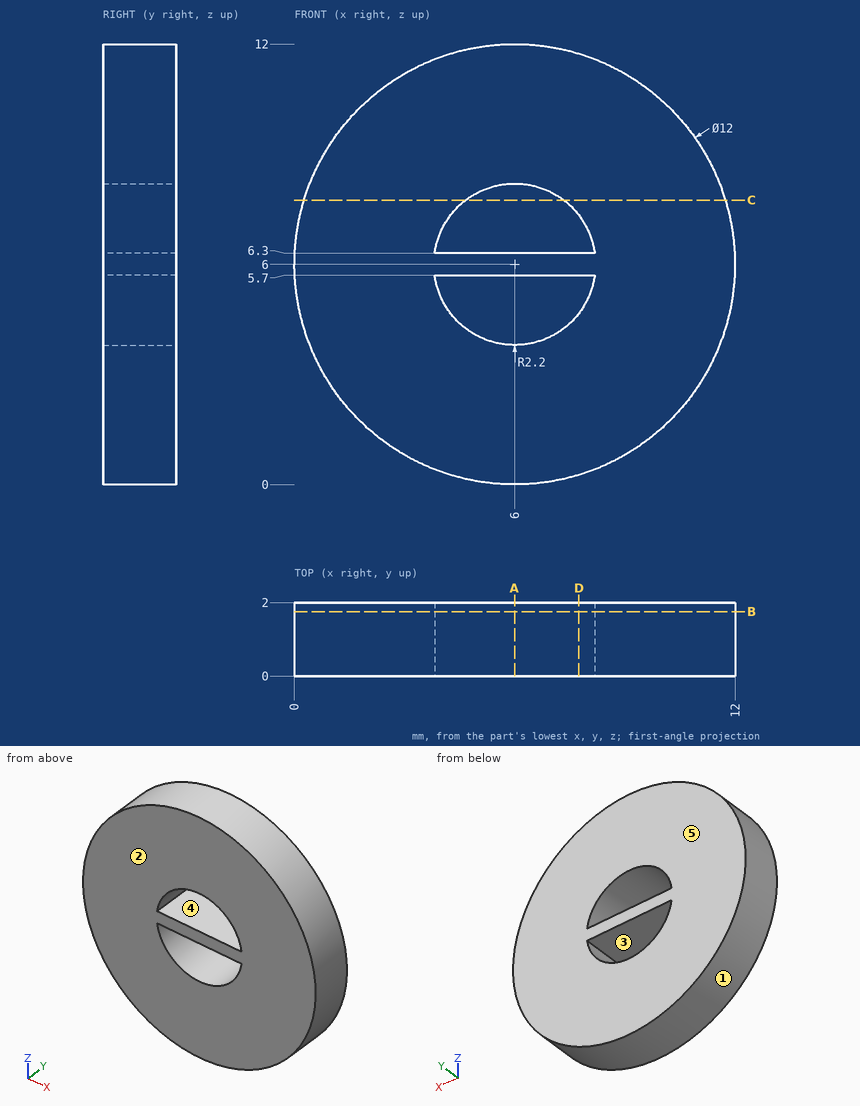
Could you check a few things on this drawing? It's one solid part, dimensions in mm from its lowest x, y, z. A direction names the side the tool comes from. Give positions to 0.01 mm unless a question says otherwise; leave off trailing zeros. Order: outer loops, then holes, each group sorted by start corner. A loop starts at its lowest first (then second) coordinate and runs counter-clockwise, first axis right, second up.
1. Which directions (+Z, -Z, +X, -X, +Y, -Y) give clear straight access to the entire face, cutting with the end or side of a thin tool? Please do the marked faces 4 and 5.
Answers below:
face 4: +Y, -Y
face 5: +Z, -Z, +X, -X, +Y
2. Suppose I cut it at C-C (z = 7.75). Write out the boundary of the cut face in (x, y).
Answers below:
outline: (0.26, 0) - (4.67, 0) - (4.67, 2) - (0.26, 2) - close; (7.33, 0) - (11.74, 0) - (11.74, 2) - (7.33, 2) - close
3. I need wall thicknesses on L1, parallel to Z at x = 4.5, y = 1.75; L2, parallel to Z at x = 6.25, y = 1.25; L3, parallel to X at y = 0.7, z = 7.75. Which ranges of each line are inside material? Lowest first, please.
Answers below:
L1: z = 0.19 to 4.39, 5.7 to 6.3, 7.61 to 11.81
L2: z = 0.01 to 3.81, 5.7 to 6.3, 8.19 to 11.99
L3: x = 0.26 to 4.67, 7.33 to 11.74
4. Suppose I cut it at B-B (y = 1.75). Write out the boundary of the cut face in (x, z).
Answers below:
outline: circle Ø12 at (6, 6); hole (3.82, 5.7) arc R2.2 ccw to (8.18, 5.7) - close; hole (3.82, 6.3) - (8.18, 6.3) arc R2.2 ccw to start
5. Suppose I cut it at A-A (x = 6). Write out the boundary of the cut face in (y, z), plus the area to 3 significant figures.
Answers below:
outline: (0, 0) - (2, 0) - (2, 3.8) - (0, 3.8) - close; (0, 5.7) - (2, 5.7) - (2, 6.3) - (0, 6.3) - close; (0, 8.2) - (2, 8.2) - (2, 12) - (0, 12) - close
area: 16.4 mm2
6. Thinking about a two-plate mould opening in Z: for the marked faces 1, 2 and 3, which applies, +Z half, -Z half, draft (parallel to the pull), parting line (faces both ways), or undercut?
Answers below:
face 1: parting line
face 2: draft
face 3: undercut
7. Suppose I cut it at D-D (x = 7.75). Write out the boundary of the cut face in (y, z).
Answers below:
outline: (0, 0.26) - (2, 0.26) - (2, 4.67) - (0, 4.67) - close; (0, 5.7) - (2, 5.7) - (2, 6.3) - (0, 6.3) - close; (0, 7.33) - (2, 7.33) - (2, 11.74) - (0, 11.74) - close
